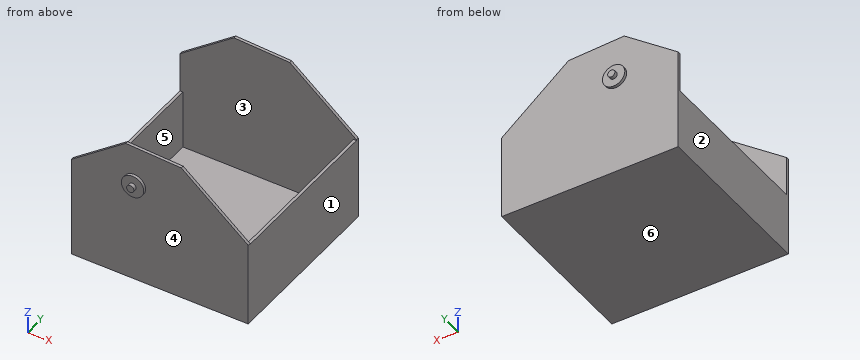
from build123d import *

# Parameters (mm, degrees)
BOSS_EXTRUDE1_DEPTH = 3.2
SKETCH3_R           = 12.3
BOSS_EXTRUDE2_DEPTH = 3.2
SKETCH4_R           = 4
BOSS_EXTRUDE3_DEPTH = 4
SKETCH6_W           = 3.2
SKETCH6_H           = 65
BOSS_EXTRUDE4_DEPTH = 190
SKETCH8_W           = 3.2
SKETCH8_H           = 89
BOSS_EXTRUDE5_DEPTH = 190
SKETCH9_W           = 194.2
SKETCH9_H           = 190
BOSS_EXTRUDE7_DEPTH = 3.2


with BuildPart() as part:
    # Sketch1 → Boss-Extrude1 (new body)
    with BuildSketch(Plane(origin=(0, 0, 0), x_dir=(1, 0, 0), z_dir=(0, 1, 0))):
        Polygon((-71.199297972, 0), (119.800702028, 0), (119.800702028, -90), (46.272924854, -150.155348756), (-15.035731115, -153.181069815), (-74.399297972, -109), (-74.399297972, -65), (-71.199297972, -65), align=None)
    boss_extrude1 = extrude(amount=BOSS_EXTRUDE1_DEPTH)

    # Sketch3 → Boss-Extrude2 (add)
    with BuildSketch(Plane.XZ):
        with Locations(Location((-5.399297972, 108.199281837, 0), (0, 0, 270))):
            Circle(SKETCH3_R)
    boss_extrude2 = extrude(amount=BOSS_EXTRUDE2_DEPTH)

    # Sketch4 → Boss-Extrude3 (add)
    with BuildSketch(Plane.XZ.offset(3.2)):
        with Locations(Location((-5.399297972, 108.199281837, 0), (0, 0, 270))):
            Circle(SKETCH4_R)
    boss_extrude3 = extrude(amount=BOSS_EXTRUDE3_DEPTH)

    # Sketch6 → Boss-Extrude4 (add)
    with BuildSketch(Plane(origin=(0, 0, 0), x_dir=(1, 0, 0), z_dir=(0, 1, 0))):
        with Locations((-72.799297972, -32.5)):
            Rectangle(SKETCH6_W, SKETCH6_H)
    extrude(amount=BOSS_EXTRUDE4_DEPTH)

    # Sketch8 → Boss-Extrude5 (add)
    with BuildSketch(Plane(origin=(0, 0, 0), x_dir=(1, 0, 0), z_dir=(0, 1, 0))):
        with Locations((118.200702028, -44.5)):
            Rectangle(SKETCH8_W, SKETCH8_H)
    extrude(amount=BOSS_EXTRUDE5_DEPTH)

    # Mirror1: Boss-Extrude1, Boss-Extrude2, Boss-Extrude3 across plane
    add(boss_extrude1.mirror(Plane(origin=(0, 95, 0), x_dir=(0, 0, 1), z_dir=(0, -1, 0))))
    add(boss_extrude2.mirror(Plane(origin=(0, 95, 0), x_dir=(0, 0, 1), z_dir=(0, -1, 0))))
    add(boss_extrude3.mirror(Plane(origin=(0, 95, 0), x_dir=(0, 0, 1), z_dir=(0, -1, 0))))

    # Sketch9 → Boss-Extrude7 (add)
    with BuildSketch(Plane.XY):
        with Locations((22.700702028, 95)):
            Rectangle(SKETCH9_W, SKETCH9_H)
    extrude(amount=-BOSS_EXTRUDE7_DEPTH)


solid = part.part
The listing builds one solid part. Answer for the finished solid, in the listing's coordinates (mm). Face numbers are marked on the shaded views. A direction names the side the tool comes from. Coordinates: 2 decimals unless noted, no trailing zeros. Loops run counter-clockwise (first coordinate to the right, second up) from the corner with the lowest first, then second, coordinate; pieces in that order, holes last. Notation, with made-up numbers: (-13.5, -24) -> (-5.5, -24) arc R31 cw to (-5.5, 2) -> close; hole circle Ø11 at (31.5, 35.5). An arc over 180 degrees is marked (long way). Answer in a Markdown table with one row per item. Add a question column.
1. The part is cut by section B-B, the plane z = 47. Write down the section's boundary in (x, y).
2. The part is cut by section A-A, the plane z = 130.5. Write down the section's boundary in (x, y), then the cut area to 3 significant figures.
3. Consider line 1 (Y direction, x = 52, z = 61.5); line 2 (X direction, y = 57.5, z = 30); line 3 (Z direction, x = 86, y = 113.5). Determine where each line is inside the solid, lowest interval first. Write a range as [from, to].
4. Determine the mould class of the marked faces 1, 2, 3 and 4 for opening direction X: +X half, -X half, draft (parallel to the pull), parting line (faces both ways), or undercut.
5. Flat-ended cylindrical pins translate along their axes: P1, Ø3, axis at x = 17.5, z = 133, coming from the -Y side; P2, Ø12, axis at x = -51.5, z = 61.5, coming from the +Y side; P3, Ø1, axis at x = -73, y = 55.5, coming from the +Z side. Find the tip coordinate at first contact, or state that the pin passes through.
6. The part is cut by section D-D, the plane x = -28. Write down the section's boundary in (y, z), then the cut area to 3 significant figures.
7. For the marked faces 5 and 6, determine the directions among +Z, -Z, +X, -X, +Y, -Y from which every point of the face is accessible in a straight line to the end or side of a thin tool.
8. The part is cut by section C-C, the plane y = 180. Write down the section's boundary in (x, z).
Answer below:
| question | item | result |
|---|---|---|
| 1 | outline | (-74.4, 0) -> (119.8, 0) -> (119.8, 190) -> (-74.4, 190) -> close; hole (-71.2, 3.2) -> (116.6, 3.2) -> (116.6, 186.8) -> (-71.2, 186.8) -> close |
| 2 | outline | (-45.51, 0) -> (70.3, 0) -> (70.3, 3.2) -> (-45.51, 3.2) -> close; (-45.51, 186.8) -> (70.3, 186.8) -> (70.3, 190) -> (-45.51, 190) -> close |
| 2 | area | 741 mm2 |
| 3 | line 1 | [0, 3.2], [186.8, 190] |
| 3 | line 2 | [-74.4, -71.2], [116.6, 119.8] |
| 3 | line 3 | [-3.2, 0] |
| 4 | face 1 | +X half |
| 4 | face 2 | -X half |
| 4 | face 3 | undercut |
| 4 | face 4 | draft |
| 5 | P1 | y = 0 |
| 5 | P2 | y = 190 |
| 5 | P3 | z = 65 |
| 6 | outline | (0, -3.2) -> (190, -3.2) -> (190, 143.53) -> (186.8, 143.53) -> (186.8, 0) -> (3.2, 0) -> (3.2, 143.53) -> (0, 143.53) -> close |
| 6 | area | 1,530 mm2 |
| 7 | face 5 | +Z |
| 7 | face 6 | -Z, +X, -X, +Y, -Y |
| 8 | outline | (-74.4, -3.2) -> (119.8, -3.2) -> (119.8, 89) -> (116.6, 89) -> (116.6, 0) -> (-71.2, 0) -> (-71.2, 65) -> (-74.4, 65) -> close |
